Check sheet for the modelled part. Datum: model origin and axes. Units: mm. A direction names the side the tool comes from. Coordinates: 2 decimals unless noted, no trailing zeros. Loops run counter-clockwise (first coordinate to the right, second up) from the corner with the lowest first, then second, coordinate; pieces in that order, holes last.
Autodesk Inventor part; units mm, degrees
ref_plane "作業平面1" through (0, 0, 11) normal (0, 0, 1) x (1, 0, 0)
ref_plane "YZ Plane" through (0, 0, 0) normal (1, 0, 0) x (0, 1, 0)
ref_plane "XZ Plane" through (0, 0, 0) normal (0, 1, 0) x (-1, 0, 0)
sketch "スケッチ1" plane through (0, 0, 0) normal (0, 0, 1) x (1, 0, 0)
  circle A0 centre (0, 0) radius 3
  circle A1 centre (0, 0) radius 1.5
  dimension "d0" = 6
  dimension "d1" = 3
extrude "押し出し1" add sketch "スケッチ1" along normal blind 17
ref_plane "作業平面1" through (0, 0, 11) normal (0, 0, 1) x (1, 0, 0)
sketch "スケッチ2" plane through (0, 0, 11) normal (0, 0, 1) x (1, 0, 0)
  circle A0 centre (0, 0) radius 1.5
  circle A1 centre (0, 0) radius 3
extrude "押し出し2" add sketch "スケッチ2" against normal blind 5 contours A0
properties part number "スペーサーm3-17　簡易筒型" material "アルミニウム 2014-T4"
1) Section check A-A on x = 0. Enter the section's corners in (y, z), plus the area to 3 significant figures.
Answer sheet:
outline: (-3, 0) - (-1.5, 0) - (-1.5, 6) - (1.5, 6) - (1.5, 0) - (3, 0) - (3, 17) - (1.5, 17) - (1.5, 11) - (-1.5, 11) - (-1.5, 17) - (-3, 17) - close
area: 66.0 mm2
2) Depth check by flat-ended pin: pin 1 (2.5 mm diameter, centred on x = 0, y = 0, fed in from -Z); pin 2 (2 mm diameter, centred on x = -1.5, z = 12, fed in from +Y); pin 3 (1.8 mm diameter, centred on x = 0, y = 0, fed in from +Z). Enter the tip coordinate at first touch or a pass-through.
Answer sheet:
pin 1: stops at z = 6
pin 2: stops at y = 2.96
pin 3: stops at z = 11
3) Scan lines: line 1 (Y direction, x = 0, z = 12.7); line 2 (Z direction, x = -0.5, y = -1); line 3 (X direction, y = 1.1, z = 2.5). Record each from-to range of solid material in increasing order.
Answer sheet:
line 1: y = -3 to -1.5, 1.5 to 3
line 2: z = 6 to 11
line 3: x = -2.79 to -1.02, 1.02 to 2.79
4) Section check B-B on z = 14. Enter the section's corners in (x, y), plus the area to 3 significant figures.
Answer sheet:
outline: circle Ø6 at (0, 0); hole circle Ø3 at (0, 0)
area: 21.2 mm2
5) Set-up check for faces 1 (the flat face through (1.3, -1.3, 17)), 2 (the cylindrical face through (-1.5, -0.07, 13.96)), 3 (the flat face through (0, 0, 6)): record each of +Z, -Z, +X, -X, +Y, -Y from which the full face is reachable in a straight line by a thin tool's end or side.
Answer sheet:
face 1: +Z, +X, -X, +Y, -Y
face 2: +Z
face 3: -Z
6) Mould release check, pull along Y, two halves, no side actions. Record for faces 4 (the cylindrical face through (-3, 0, 8)), 5 (the flat face through (0, 0, 11)), 6 (the flat face through (1.3, -1.3, 0)): +Y half, -Y half, draft (parallel to the pull), parting line (faces both ways), or undercut.
Answer sheet:
face 4: parting line
face 5: undercut
face 6: draft
7) Section check D-D on z = 7. Enter the section's corners in (x, y), plus the area to 3 significant figures.
Answer sheet:
outline: circle Ø6 at (0, 0)
area: 28.3 mm2
